Geometry: final body of the model. Coordinates: model frame, mm. Face numbers are marked on the shaded views. A direction names the side the tool comes from. Coordinates: 2 decimals unless noted, no trailing zeros. Loops run counter-clockwise (first coordinate to the right, second up) from the corner with the lowest first, then second, coordinate; pieces in that order, holes last. Notation, with made-up numbers: (25.5, 8) -> (61.5, 8) arc R18 ccw to (61.5, 42) -> close; hole circle Ø9 at (-25, 52). An arc over 180 degrees is marked (long way). One line per item, written item: value. Start each with the question number.
Item 1: Ray query, probe 1 along X at (y, z) = (23.25, 10.25); probe 2 along Z at (x, y) = (31, 26.5); probe 3 along X at (y, z) = (4.25, 8). Return the intervals inside material, ascending. Write a range as from..to.
Item 2: Section query B-B on x = 27. Return loops of the section in (y, z).
Item 3: Section query C-C on y = 26. Return loops of the section in (x, z), then the cut area to 3 significant figures.
Item 4: Section query A-A on z = 13. Return loops of the section in (x, y).
Item 5: Mould query, pull axis Z, two halves, no side actions, for the marked faces 1, 2, 3 and 4. Classes: +Z half, -Z half, draft (parallel to the pull), parting line (faces both ways), or undercut.
Item 6: Contact query for flat-ended pins moving along their axis: pin 1 Ø9.5 at (x, y) = (49, 25) entering from +Z; pin 2 Ø4 at (x, y) = (53.5, 9.5) entering from +Z; pin 3 Ø2 at (x, y) = (30.5, 9.5) entering from +Z. Output: stop coordinate, or through.
Item 7: Section query D-D on z = 4.25. Return loops of the section in (x, y), then the cut area to 3 significant figures.
Item 8: Set-up query: the marked faces 5, 6 and 7. Return all of +Z, -Z, +X, -X, +Y, -Y with unobstructed straight access to the full face (end or side cutting, diameter ignored); none if empty.
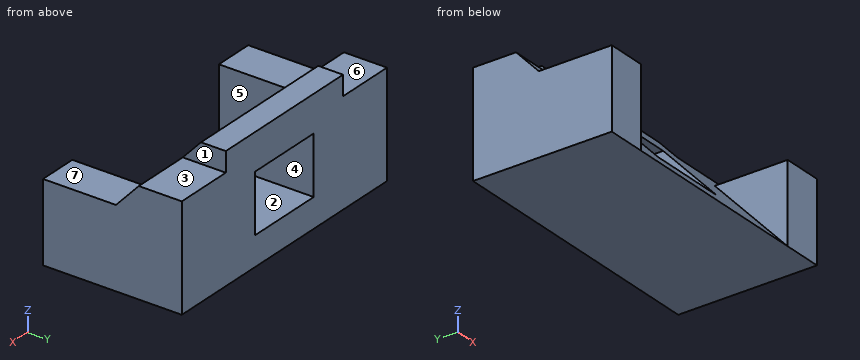
Autodesk Fusion 360 part; units mm, degrees
sketch "Sketch1" plane through (0, 0, 0) normal (0, 0, 1) x (1, 0, 0)
box "BoxPrimitive1" add length 28 width 56 height 25 placed x (0, 1, 0) y (-1, 0, 0) z (0, 0, 1) at (56, 0, 0)
sketch "Sketch2" plane through (56, 0, 0) normal (1, 0, 0) x (0, 1, 0)
  line L0 (0, 25) -> (0, 0)
  line L1 (0, 0) -> (28, 0)
  line L2 (28, 0) -> (28, 25)
  line L3 (28, 25) -> (0, 25)
  line L4 (0, 0) -> (23, 25)
  line L5 (28, 21) -> (19.32, 21)
  line L6 (0, 16) -> (14.72, 16)
  dimension "d6" = 5
  dimension "d7" = 16
  dimension "d8" = 5
extrude "Extrude1" cut sketch "Sketch2" against normal blind 56 contours L0 L3 L4 L6
extrude "Extrude2" cut sketch "Sketch2" against normal blind 40 from surface at -8 contours L0 L4 L6
extrude "Extrude3" cut sketch "Sketch2" against normal blind 12 contours L2 L3 L4 L5
ref_plane "WorkPlane1" through (28, 14, 12.5) normal (-1, 0, 0) x (0, 0, 1)
mirror "Mirror1" about plane through (28, 14, 12.5) normal (-1, 0, 0) of "Extrude3"
sketch "Sketch3" plane through (0, 0, 0) normal (0, -0.7359, 0.6771) x (1, 0, 0)
  line L0 (12, 28.5353) -> (0, 28.5353)
  line L1 (0, 28.5353) -> (0, 21.7412)
  line L2 (0, 21.7412) -> (8, 21.7412)
  line L3 (8, 21.7412) -> (8, 0)
  line L4 (8, 0) -> (48, 0)
  line L5 (48, 0) -> (48, 21.7412)
  line L6 (48, 21.7412) -> (56, 21.7412)
  line L7 (56, 21.7412) -> (56, 28.5353)
  line L8 (56, 28.5353) -> (44, 28.5353)
  line L9 (44, 28.5353) -> (44, 33.9706)
  line L10 (44, 33.9706) -> (12, 33.9706)
  line L11 (12, 33.9706) -> (12, 28.5353)
  line L12 (20, 24) -> (36, 24)
  line L13 (36, 24) -> (36, 8)
  line L14 (36, 8) -> (20, 8)
  line L15 (20, 8) -> (20, 24)
  dimension "d18" = 16
  dimension "d19" = 16
  dimension "d20" = 8
  dimension "d21" = 12
sketch "Sketch4" plane through (0, 28, 0) normal (0, 1, 0) x (-1, 0, 0)
  line L0 (0, 21) -> (-12, 21)
  line L1 (-12, 21) -> (-12, 25)
  line L2 (-12, 25) -> (-44, 25)
  line L3 (-44, 25) -> (-44, 21)
  line L4 (-44, 21) -> (-56, 21)
  line L5 (-56, 21) -> (-56, 0)
  line L6 (-56, 0) -> (0, 0)
  line L7 (0, 0) -> (0, 21)
  line L8 (-36, 5.8874) -> (-20, 5.8874)
  line L9 (-20, 5.8874) -> (-20, 17.6623)
  line L10 (-36, 17.6623) -> (-36, 5.8874)
  line L11 (-20, 17.6623) -> (-36, 17.6623)
extrude "Extrude4" cut sketch "Sketch4" against normal blind 28 contours L8 L9 L10 L11
Reply:
1. probe 1: x = 0..20, 36..56
1. probe 2: z = 0..5.89, 17.66..25
1. probe 3: x = 0..8, 48..56
2. outline: (0, 0) -> (28, 0) -> (28, 5.89) -> (5.42, 5.89) -> close; (16.25, 17.66) -> (28, 17.66) -> (28, 25) -> (23, 25) -> close
3. outline: (0, 0) -> (56, 0) -> (56, 21) -> (44, 21) -> (44, 25) -> (12, 25) -> (12, 21) -> (0, 21) -> close; hole (20, 5.89) -> (36, 5.89) -> (36, 17.66) -> (20, 17.66) -> close
3. area: 1,120 mm²
4. outline: (0, 0) -> (8, 0) -> (8, 11.96) -> (20, 11.96) -> (20, 28) -> (0, 28) -> close; (36, 11.96) -> (48, 11.96) -> (48, 0) -> (56, 0) -> (56, 28) -> (36, 28) -> close
5. face 1: draft
5. face 2: undercut
5. face 3: +Z half
5. face 4: undercut
6. pin 1: stops at z = 21
6. pin 2: stops at z = 16
6. pin 3: stops at z = 5.89
7. outline: (0, 0) -> (8, 0) -> (8, 3.91) -> (48, 3.91) -> (48, 0) -> (56, 0) -> (56, 28) -> (0, 28) -> close
7. area: 1,410 mm²
8. face 5: +Z, -Y
8. face 6: +Z, -X, +Y, -Y
8. face 7: +Z, +X, -X, -Y
